Autodesk Inventor part; units mm, degrees
ref_plane "Work Plane2" through (0, 1, 0) normal (0, -1, 0) x (1, 0, 0)
ref_plane "Work Plane3" through (8, 0, 0) normal (1, 0, 0) x (0, 1, 0)
ref_plane "XZ Plane" through (0, 0, 0) normal (0, 1, 0) x (-1, 0, 0)
sketch "Sketch1" plane through (0, 0, 0) normal (0, 1, 0) x (-1, 0, 0)
  circle A0 centre (0, 0) radius 10
  circle A1 centre (0, 0) radius 26
  dimension "d0" = 20
  dimension "d8" = 52
extrude "Extrusion1" add sketch "Sketch1" along normal blind 5
sketch "Sketch2" plane through (0, 0, 0) normal (0, -1, 0) x (1, 0, 0)
  circle A0 centre (0, 0) radius 14
  circle A1 centre (0, 0) radius 10
  dimension "d56" = 28
extrude "Extrusion2" add sketch "Sketch2" along normal blind 2.5
sketch "Sketch3" plane through (0, 5, 0) normal (0, 1, 0) x (1, 0, 0)
  circle A0 centre (0, 0) radius 21 construction
  line L0 (36.4, 0) -> (-36.4, 0)
  circle A1 centre (0, 0) radius 21 construction
  circle A2 centre (0, 0) radius 21 construction
  point P0 (-21, 0)
  point P1 (10.5, -18.1865)
  point P2 (10.5, 18.1865)
  dimension "d7" = 42
  dimension "d11" = 360
hole "Hole1" at (-21, 5, 0) at (10.5, 5, 18.1865) at (10.5, 5, -18.1865) direction (0, -1, 0) diameter 3.4 end through all counterbore diameter 6.5 counterbore depth 3.4
ref_plane "Work Plane2" through (0, 1, 0) normal (0, -1, 0) x (1, 0, 0)
sketch "Sketch8" plane through (0, 1, 0) normal (0, -1, 0) x (1, 0, 0)
  circle A0 centre (0, 0) radius 10
  circle A1 centre (0, 0) radius 10
  circle A2 centre (0, 0) radius 3
  dimension "d39" = 6
extrude "Extrusion5" add sketch "Sketch8" against normal blind 9
ref_plane "Work Plane3" through (8, 0, 0) normal (1, 0, 0) x (0, 1, 0)
sketch "Sketch9" plane through (0, 10, 0) normal (0, 1, 0) x (1, 0, 0)
  circle A0 centre (0, 0) radius 8
  circle A1 centre (0, 0) radius 3
  circle A2 centre (0, 0) radius 10
  circle A3 centre (0, 0) radius 3
  dimension "d43" = 5
extrude "Extrusion6" cut sketch "Sketch9" against normal blind 5 contours A2
sketch "Sketch10" plane through (8, 0, 0) normal (1, 0, 0) x (0, 1, 0)
  line L0 (5, -8) -> (5, 8)
  line L1 (10, -8) -> (10, 8)
  line L2 (10, 0) -> (5, 0) construction
  point P0 (0, 0)
  point P1 (7.5, 0)
hole "Hole3" at (8, 7.5, 0) direction (-1, 0, 0) diameter 2.459 depth 8.8 tip angle 118
chamfer "Chamfer1" distance 0.5 angle 45 1 edges at (-14, -2.5, 0)
properties part number "rotation stopper"
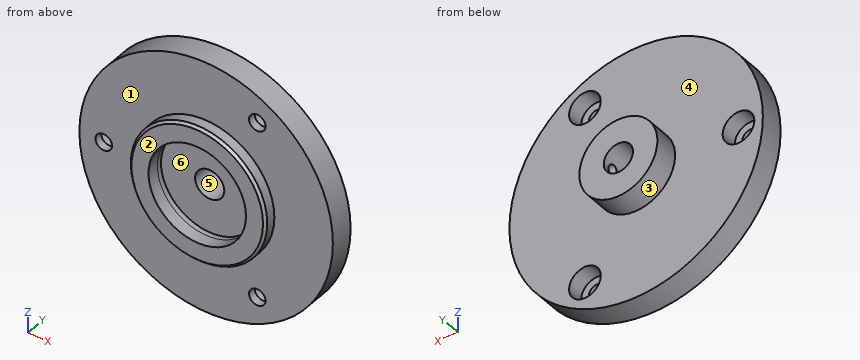
Part model, mm, in its own coordinate system. Face numbers are marked on the shaded views. A direction names the side the tool comes from. Give positions to 0.01 mm unless a question says otherwise; leave off trailing zeros. Write each loop counter-clockwise with the first axis right and the second up, starting at its lowest first coordinate (ties: lowest second). Pieces come first, ordered by that corner, then holes. Notation, with made-up numbers: M 11,47.5 L 68,47.5 A33 cw 68,76.5 Z; hole C 78,-31.5 d2. An arc over 180 degrees is marked long. Use CSV: the item, a comma, the result in double quotes.
Item 1: Slice it at B-B on x = 0. Write the cut outline in (y, z), plus the area to 3 significant figures.
Taken from the geometry:
outline,"M -2.5,-13.5 L -2,-14 L 0,-14 L 0,-26 L 5,-26 L 5,-8 L 10,-8 L 10,-3 L 1,-3 L 1,-10 L -2.5,-10 Z; M -2.5,10 L 1,10 L 1,3 L 10,3 L 10,8 L 5,8 L 5,26 L 0,26 L 0,14 L -2,14 L -2.5,13.5 Z"
area,"286 mm²"
Item 2: Drill centre lines: probe 1 along Z at (x, y) = (9, 0.75); probe 2 along Z at (x, y) = (10.5, 3.15); probe 3 along Y at (x, z) = (7, 15.5). Where is each one in solid material? Low to high.
Taken from the geometry:
probe 1,"z = -24.39 to -18.99, -17.39 to -4.36, 4.36 to 17.39, 18.99 to 24.39"
probe 2,"z = -23.79 to -21.44, -14.94 to 14.94, 21.44 to 23.79"
probe 3,"y = 0 to 5"
Item 3: Slice it at D-D on y = -0.75. Write the cut outline in (x, z), plus the area to 3 significant figures.
Taken from the geometry:
outline,"C 0,0 d28; hole C 0,0 d20"
area,"302 mm²"
Item 4: Which spindle directions (+Z, -Z, +X, -X, +Y, -Y) get a long thin tool onto all of the face, cutting with end or side? Do the marked faces 1 and 2. Say none if no direction does.
Taken from the geometry:
face 1,"-Y"
face 2,"+Z, -Z, +X, -X, -Y"
Item 5: Slice it at A-A on z = 0. State how many separate pieces and enclosed holes the cut face has, plus the area to 3 significant figures.
Taken from the geometry:
separate pieces,"4"
enclosed holes,"0"
area,"246 mm²"
Item 6: Slice it at C-C on y = 2.5. Write the cut outline in (x, z).
Taken from the geometry:
outline,"C 0,0 d52; hole C -21,0 d6.5; hole C 0,0 d6; hole C 10.5,-18.19 d6.5; hole C 10.5,18.19 d6.5"
Item 7: Pull direction Z, two halves, no side cores. Call the marked faces 3, 4, 5 and 6: +Z half, -Z half, draft (parallel to the pull), parting line (faces both ways), or undercut.
Taken from the geometry:
face 3,"parting line"
face 4,"draft"
face 5,"undercut"
face 6,"undercut"
Item 8: Pin check, flat tips, straight feed: P1, Ø10.5, axis at x = 10.5, z = 18.19, coming from the -Y side; P2, Ø5, axis at x = 12, z = -18.5, coming from the +Y side; P3, Ø23, axis at x = 0, z = 0, coming from the -Y side; P4, Ø2, axis at x = 18.5, y = 2, coming from the -Z side. Stop position of each tip, or through.
Taken from the geometry:
P1,"stops at y = 0"
P2,"stops at y = 5"
P3,"stops at y = -2.5"
P4,"stops at z = -19.23"
